Here's how the part is built. I have some questions about the finished solid (model axes, mm). A direction names the side the tool comes from. Round coordinates to 2 decimals unless told otherwise and drop trailing zeros. Order: outer loops, then holes, each group sorted by start corner. A loop starts at its lowest first (then second) coordinate and runs counter-clockwise, first axis right, second up. Notation, with made-up numbers: M 86,79 L 111,79 A32 cw 111,108 Z; hole C 48,-1 d11. An arc over 180 degrees is marked long. Write item = value, one per line. Start each with the question number.
Item 1: I want a section at A-A, the plane x = 1. List the corners of the cut face in (y, z) for me.
Item 2: I'm going to push flat-ended pins straight in: P1, Ø6, axis at y = 21, z = 26, coming from the +X side; P2, Ø1, axis at x = -18.5, z = 27.5, coming from the +Y side; P3, Ø3.5, axis at x = 10, y = -6, coming from the +Z side. Where does each tip first touch, or does it pass through?
Item 3: Please list where these lines run through material, in increasing order: L1, parallel to X at y = -9, z = 71.5; L2, parallel to X at y = -9, z = 5; L3, parallel to X at y = 28.5, z = 10.5.
Item 4: I want a section at B-B, the plane y = -8.5. State how many separate pieces and enclosed holes the cut face has, plus the area to 3 significant figures.
Item 5: We'd pull the mould along Z, two halves only. Please class faces 4 (the face through (14.584, -6.699, 34.894)), 5 (the face through (18, -6, 20.333)), 6 (the face through (21, -12, 4)), 7 (the face through (-9, -8, 81.333)): pulls with the +Z half, pulls with the -Z half, needs draft (parallel to the pull), parting line crosses it, or undercut.
Item 6: I want a section at D-D, the plane x = -27.5. List the corners of the cut face in (y, z) for me, plus the area to 3 significant figures.
Item 7: I want a section at C-C, the plane y = 26.5. List the corners of the cut face in (x, z) for me, plus the area to 3 significant figures.
Item 8: For faces 1 (the face through (-19, -6, 18.833)), 2 (the face through (-18, -12, 25)), 3 (the face through (17.804, -6.177, 14.561)), which set-ups out of +Z, -Z, +X, -X, +Y, -Y let a thin tool reach every point of the face, with its end or its side?
```python
from build123d import *

# Parameters (mm, degrees)
F1_DEPTH     = 12
F3_DEPTH     = 40
F5_DEPTH     = 5
F6_W         = 38
F6_H         = 100.4237157875
F7_DEPTH     = 7.5
F9_DEPTH     = 7.5
F10_T4_DEPTH = 100.2951088773
F10_T9_DEPTH = 100.2951088773
F11_R        = 20


# Not quite as in the source:
# - a fillet or chamfer that OpenCascade refuses, or shapes differently, is made with other operations: its cross-section is extruded or revolved along the edge and cut away or added


with BuildPart() as f1:
    # F0 (on Front) → F1 (new body)
    with BuildSketch(Plane.XZ):
        Polygon((-18.7375766605, 8.6666666667), (-21.7375766605, 8.6666666667), (-23.11024181, 0), (-20.11024181, 0), align=None)
    extrude(amount=F1_DEPTH)


with BuildPart() as f1b:
    # F0 (on Front) → F1, piece 2 (new body)
    with BuildSketch(Plane.XZ):
        Polygon((21.7375766605, 8.6666666667), (18.7375766605, 8.6666666667), (20.11024181, 0), (23.11024181, 0), align=None)
    extrude(amount=F1_DEPTH)


with BuildPart() as f1c:
    # F0 (on Front) → F1, piece 3 (new body)
    with BuildSketch(Plane.XZ):
        Polygon((-20.1273348505, 18.8333333333), (-21.5, 10.1666666667), (-18.5, 10.1666666667), (-17.1273348505, 18.8333333333), align=None)
    extrude(amount=F1_DEPTH)


with BuildPart() as f1d:
    # F0 (on Front) → F1, piece 4 (new body)
    with BuildSketch(Plane.XZ):
        Polygon((17.1273348505, 18.8333333333), (18.5, 10.1666666667), (21.5, 10.1666666667), (20.1273348505, 18.8333333333), align=None)
    extrude(amount=F1_DEPTH)


with BuildPart() as f1e:
    # F0 (on Front) → F1, piece 5 (new body)
    with BuildSketch(Plane.XZ):
        Polygon((-15.5170930406, 29), (-18.5170930406, 29), (-19.88975819, 20.3333333333), (-16.88975819, 20.3333333333), align=None)
    extrude(amount=F1_DEPTH)


with BuildPart() as f1f:
    # F0 (on Front) → F1, piece 6 (new body)
    with BuildSketch(Plane.XZ):
        Polygon((16.88975819, 20.3333333333), (19.88975819, 20.3333333333), (18.5170930406, 29), (15.5170930406, 29), align=None)
    extrude(amount=F1_DEPTH)


with BuildPart() as f1g:
    # F0 (on Front) → F1, piece 7 (new body)
    with BuildSketch(Plane.XZ):
        Polygon((-15.2966094206, 49.3333333333), (-16.6692745701, 40.6666666667), (-13.6692745701, 40.6666666667), (-12.2966094206, 49.3333333333), align=None)
    extrude(amount=F1_DEPTH)


with BuildPart() as f1h:
    # F0 (on Front) → F1, piece 8 (new body)
    with BuildSketch(Plane.XZ):
        Polygon((-10.6863676107, 59.5), (-13.6863676107, 59.5), (-15.0590327601, 50.8333333333), (-12.0590327601, 50.8333333333), align=None)
    extrude(amount=F1_DEPTH)


with BuildPart() as f1i:
    # F0 (on Front) → F1, piece 9 (new body)
    with BuildSketch(Plane.XZ):
        Polygon((-11.8385491402, 71.1666666667), (-8.8385491402, 71.1666666667), (-7.4658839907, 79.8333333333), (-10.4658839907, 79.8333333333), align=None)
    extrude(amount=F1_DEPTH)


with BuildPart() as f1j:
    # F0 (on Front) → F1, piece 10 (new body)
    with BuildSketch(Plane.XZ):
        Polygon((-5.8556421808, 90), (-8.8556421808, 90), (-10.2283073302, 81.3333333333), (-7.2283073302, 81.3333333333), align=None)
    extrude(amount=F1_DEPTH)


with BuildPart() as f1k:
    # F0 (on Front) → F1, piece 11 (new body)
    with BuildSketch(Plane.XZ):
        Polygon((-4.2454003708, 100.1666666667), (-7.2454003708, 100.1666666667), (-8.6180655203, 91.5), (-5.6180655203, 91.5), align=None)
    extrude(amount=F1_DEPTH)


with BuildPart() as f1l:
    # F0 (on Front) → F1, piece 12 (new body)
    with BuildSketch(Plane.XZ):
        Polygon((16.9068512306, 39.1666666667), (13.9068512306, 39.1666666667), (15.2795163801, 30.5), (18.2795163801, 30.5), align=None)
    extrude(amount=F1_DEPTH)


with BuildPart() as f1m:
    # F0 (on Front) → F1, piece 13 (new body)
    with BuildSketch(Plane.XZ):
        Polygon((15.2966094206, 49.3333333333), (12.2966094206, 49.3333333333), (13.6692745701, 40.6666666667), (16.6692745701, 40.6666666667), align=None)
    extrude(amount=F1_DEPTH)


with BuildPart() as f1n:
    # F0 (on Front) → F1, piece 14 (new body)
    with BuildSketch(Plane.XZ):
        Polygon((13.6863676107, 59.5), (10.6863676107, 59.5), (12.0590327601, 50.8333333333), (15.0590327601, 50.8333333333), align=None)
    extrude(amount=F1_DEPTH)


with BuildPart() as f1o:
    # F0 (on Front) → F1, piece 15 (new body)
    with BuildSketch(Plane.XZ):
        Polygon((10.4487909502, 61), (13.4487909502, 61), (12.0761258007, 69.6666666667), (9.0761258007, 69.6666666667), align=None)
    extrude(amount=F1_DEPTH)


with BuildPart() as f1p:
    # F0 (on Front) → F1, piece 16 (new body)
    with BuildSketch(Plane.XZ):
        Polygon((10.4658839907, 79.8333333333), (7.4658839907, 79.8333333333), (8.8385491402, 71.1666666667), (11.8385491402, 71.1666666667), align=None)
    extrude(amount=F1_DEPTH)


with BuildPart() as f1q:
    # F0 (on Front) → F1, piece 17 (new body)
    with BuildSketch(Plane.XZ):
        Polygon((8.8556421808, 90), (5.8556421808, 90), (7.2283073302, 81.3333333333), (10.2283073302, 81.3333333333), align=None)
    extrude(amount=F1_DEPTH)


with BuildPart() as f1r:
    # F0 (on Front) → F1, piece 18 (new body)
    with BuildSketch(Plane.XZ):
        Polygon((-13.9068512306, 39.1666666667), (-16.9068512306, 39.1666666667), (-18.2795163801, 30.5), (-15.2795163801, 30.5), align=None)
    extrude(amount=F1_DEPTH)


with BuildPart() as f1s:
    # F0 (on Front) → F1, piece 19 (new body)
    with BuildSketch(Plane.XZ):
        Polygon((-12.0761258007, 69.6666666667), (-13.4487909502, 61), (-10.4487909502, 61), (-9.0761258007, 69.6666666667), align=None)
    extrude(amount=F1_DEPTH)


with BuildPart() as f1t:
    # F0 (on Front) → F1, piece 20 (new body)
    with BuildSketch(Plane.XZ):
        Polygon((7.2454003708, 100.1666666667), (4.2454003708, 100.1666666667), (5.6180655203, 91.5), (8.6180655203, 91.5), align=None)
    extrude(amount=F1_DEPTH)


with BuildPart() as f1u:
    # F0 (on Front) → F1, piece 21 (new body)
    with BuildSketch(Plane.XZ):
        Polygon((-29.11024181, 0), (-13.2454003708, 100.1666666667), (-16.2454003708, 100.1666666667), (-32.11024181, 0), align=None)
    extrude(amount=F1_DEPTH)


with BuildPart() as f1v:
    # F0 (on Front) → F1, piece 22 (new body)
    with BuildSketch(Plane.XZ):
        Polygon((16.2454003708, 100.1666666667), (13.2454003708, 100.1666666667), (29.11024181, 0), (32.11024181, 0), align=None)
    extrude(amount=F1_DEPTH)


with BuildPart() as f3_tool:
    # F2 (on Right) → F3 (new body, symmetric)
    with BuildSketch(Plane.YZ):
        Polygon((-5.0742244334, 100.1666666667), (0, 0), (0, 100.1666666667), align=None)
    extrude(amount=F3_DEPTH, both=True)


with BuildPart() as f1_1:
    add(f1.part)

    # F3: cut by f3_tool
    add(f3_tool.part, mode=Mode.SUBTRACT)



with BuildPart() as f1b_1:
    add(f1b.part)

    # F3: cut by f3_tool
    add(f3_tool.part, mode=Mode.SUBTRACT)


with BuildPart() as f1c_1:
    add(f1c.part)

    # F3: cut by f3_tool
    add(f3_tool.part, mode=Mode.SUBTRACT)


with BuildPart() as f1d_1:
    add(f1d.part)

    # F3: cut by f3_tool
    add(f3_tool.part, mode=Mode.SUBTRACT)


with BuildPart() as f1e_1:
    add(f1e.part)

    # F3: cut by f3_tool
    add(f3_tool.part, mode=Mode.SUBTRACT)


with BuildPart() as f1f_1:
    add(f1f.part)

    # F3: cut by f3_tool
    add(f3_tool.part, mode=Mode.SUBTRACT)


with BuildPart() as f1g_1:
    add(f1g.part)

    # F3: cut by f3_tool
    add(f3_tool.part, mode=Mode.SUBTRACT)


with BuildPart() as f1h_1:
    add(f1h.part)

    # F3: cut by f3_tool
    add(f3_tool.part, mode=Mode.SUBTRACT)


with BuildPart() as f1i_1:
    add(f1i.part)

    # F3: cut by f3_tool
    add(f3_tool.part, mode=Mode.SUBTRACT)


with BuildPart() as f1j_1:
    add(f1j.part)

    # F3: cut by f3_tool
    add(f3_tool.part, mode=Mode.SUBTRACT)


with BuildPart() as f1k_1:
    add(f1k.part)

    # F3: cut by f3_tool
    add(f3_tool.part, mode=Mode.SUBTRACT)


with BuildPart() as f1l_1:
    add(f1l.part)

    # F3: cut by f3_tool
    add(f3_tool.part, mode=Mode.SUBTRACT)


with BuildPart() as f1m_1:
    add(f1m.part)

    # F3: cut by f3_tool
    add(f3_tool.part, mode=Mode.SUBTRACT)


with BuildPart() as f1n_1:
    add(f1n.part)

    # F3: cut by f3_tool
    add(f3_tool.part, mode=Mode.SUBTRACT)


with BuildPart() as f1o_1:
    add(f1o.part)

    # F3: cut by f3_tool
    add(f3_tool.part, mode=Mode.SUBTRACT)


with BuildPart() as f1p_1:
    add(f1p.part)

    # F3: cut by f3_tool
    add(f3_tool.part, mode=Mode.SUBTRACT)


with BuildPart() as f1q_1:
    add(f1q.part)

    # F3: cut by f3_tool
    add(f3_tool.part, mode=Mode.SUBTRACT)


with BuildPart() as f1r_1:
    add(f1r.part)

    # F3: cut by f3_tool
    add(f3_tool.part, mode=Mode.SUBTRACT)


with BuildPart() as f1s_1:
    add(f1s.part)

    # F3: cut by f3_tool
    add(f3_tool.part, mode=Mode.SUBTRACT)


with BuildPart() as f1t_1:
    add(f1t.part)

    # F3: cut by f3_tool
    add(f3_tool.part, mode=Mode.SUBTRACT)


with BuildPart() as f1u_1:
    add(f1u.part)

    # F3: cut by f3_tool
    add(f3_tool.part, mode=Mode.SUBTRACT)


with BuildPart() as f1v_1:
    add(f1v.part)

    # F3: cut by f3_tool
    add(f3_tool.part, mode=Mode.SUBTRACT)


with BuildPart() as f1_2:
    add(f1_1.part)

    add(f1b_1.part)  # F5 merges F1b

    add(f1c_1.part)  # F5 merges F1c

    add(f1d_1.part)  # F5 merges F1d

    add(f1e_1.part)  # F5 merges F1e

    add(f1f_1.part)  # F5 merges F1f

    add(f1g_1.part)  # F5 merges F1g

    add(f1h_1.part)  # F5 merges F1h

    add(f1i_1.part)  # F5 merges F1i

    add(f1j_1.part)  # F5 merges F1j

    add(f1k_1.part)  # F5 merges F1k

    add(f1l_1.part)  # F5 merges F1l

    add(f1m_1.part)  # F5 merges F1m

    add(f1n_1.part)  # F5 merges F1n

    add(f1o_1.part)  # F5 merges F1o

    add(f1p_1.part)  # F5 merges F1p

    add(f1q_1.part)  # F5 merges F1q

    add(f1r_1.part)  # F5 merges F1r

    add(f1s_1.part)  # F5 merges F1s

    add(f1t_1.part)  # F5 merges F1t

    add(f1u_1.part)  # F5 merges F1u

    add(f1v_1.part)  # F5 merges F1v
    # F4 (on face) → F5 (join)
    with BuildSketch(Plane(origin=(0, 0, 0), x_dir=(-1, 0, 0), z_dir=(0, 0.9987193572, 0.0505929401))):
        Polygon((16.2454003708, 100.2951088773), (-16.2454003708, 100.2951088773), (-32.11024181, 0), (32.11024181, 0), align=None)
    extrude(amount=F5_DEPTH)

    # F6 (on Right) → F7 (join, symmetric)
    with BuildSketch(Plane.YZ):
        with Locations((19, 50.2118578937)):
            Rectangle(F6_W, F6_H)
    extrude(amount=F7_DEPTH, both=True)

    # F8 (on Right) → F9 (join, symmetric)
    with BuildSketch(Plane.YZ):
        Polygon((0.7220453882, 99.8437014869), (0, 100.4237157875), (-0.0806276475, 100.4196313671), (-0.4271789039, 99.9818352512), (-0.1710176838, 98.3370152763), align=None)
    extrude(amount=F9_DEPTH, both=True)

    # F10: fillet of radius 5 on 2 edges, made by hand


with BuildPart() as f10_tool2:
    # F10_s3 → F10_t4 (new body)
    with BuildSketch(Plane(origin=(0, 0, 0), x_dir=(1, 0, 0), z_dir=(0, -0.0505929401, 0.9987193572))):
        with BuildLine():
            ThreePointArc((12.5, 5), (8.9644660941, 6.4644660941), (7.5, 10))
            Line((7.5, 10), (7.5, 5))
            Line((7.5, 5), (12.5, 5))
        make_face()
    extrude(amount=F10_T4_DEPTH)

    split(bisect_by=Plane.XY.offset(100.4237157875), keep=Keep.BOTTOM)


with BuildPart() as f1_3:
    add(f1_2.part)

    # F10_t1: union F10_tool2
    add(f10_tool2.part)


with BuildPart() as f10_tool7:
    # F10_s8 → F10_t9 (new body)
    with BuildSketch(Plane(origin=(0, -5.0742244334, 100.1666666667), x_dir=(1, 0, 0), z_dir=(0, 0.0505929401, -0.9987193572))):
        with BuildLine():
            ThreePointArc((-7.5, -10), (-8.9644660941, -6.4644660941), (-12.5, -5))
            Line((-12.5, -5), (-7.5, -5))
            Line((-7.5, -5), (-7.5, -10))
        make_face()
    extrude(amount=F10_T9_DEPTH)

    split(bisect_by=Plane.XY.offset(100.4237157875), keep=Keep.BOTTOM)


with BuildPart() as f1_4:
    add(f1_3.part)

    # F10_t6: union F10_tool7
    add(f10_tool7.part)

    # F11
    f11_edges = [f1_4.edges().sort_by_distance(p)[0] for p in [
        (0, 38, 100.423716),
        (0, 38, 0),
    ]]
    fillet(f11_edges, radius=F11_R)


solid = f1_4.part
```
Filled in:
q1.outline = M -5.07,100.17 L 0,0 L 18,0 A20 ccw 38,20 L 38,80.42 A20 ccw 18,100.42 L 0,100.42 Z
q2.P1 = 7.5
q2.P2 = 3.64
q2.P3 = 100.21
q3.L1 = -20.79 to -17.79, -11.79 to -8.79, 8.79 to 11.79, 17.79 to 20.79
q3.L2 = -31.32 to -28.32, -22.32 to -19.32, 19.32 to 22.32, 28.32 to 31.32
q3.L3 = -7.5 to 7.5
q4.separate_pieces = 22
q4.enclosed_holes = 0
q4.area = 1,120 mm^2
q5.face_4 = pulls with the -Z half
q5.face_5 = undercut
q5.face_6 = needs draft
q5.face_7 = undercut
q6.outline = M -12,10.17 L -0.52,10.17 L 0,0 L 4.99,0.25 L 3.52,29.36 L -1.47,29.11 L -12,29.11 Z
q6.area = 354 mm^2
q7.outline = M -7.5,1.9 L 7.5,1.9 L 7.5,98.53 L -7.5,98.53 Z
q7.area = 1,450 mm^2
q8.face_1 = -Y
q8.face_2 = +Z, -Z, +X, -X, -Y
q8.face_3 = -Z, -Y
